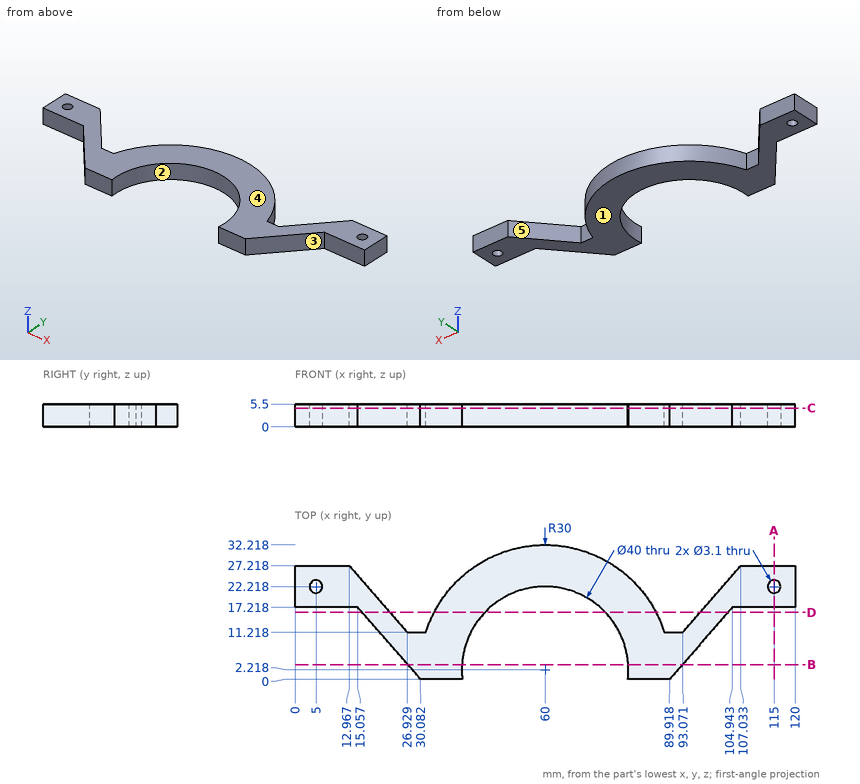
Drawing for the job (mm, zero at the part's lowest x, y, z). A direction names the side the tool comes from. Round coordinates to 2 decimals unless told otherwise and drop trailing zeros. Write each loop counter-clockwise with the first axis right and the second up, starting at its lowest first coordinate (ties: lowest second). Pieces come first, ordered by that corner, then holes. Notation, with made-up numbers: M 83,-21 L 105,-21 A21 ccw 105,7 Z; hole C -15.5,-6.5 d5. An arc over 180 degrees is marked long. One line per question, with ' | ' between items.
1. Cut at A-A on x = 115. Write the cut outline in (y, z).
Working result:
outline: M 17.22,0 L 20.67,0 L 20.67,5.5 L 17.22,5.5 Z; M 23.77,0 L 27.22,0 L 27.22,5.5 L 23.77,5.5 Z
2. Cut at B-B on y = 3.5. Write the cut outline in (x, z), and give its area (3 significant figures).
Working result:
outline: M 27.03,0 L 40.04,0 L 40.04,5.5 L 27.03,5.5 Z; M 79.96,0 L 92.97,0 L 92.97,5.5 L 79.96,5.5 Z | area: 143 mm2
3. Mould opens along X. For the marked faces 1, 2 and 3 say: pulls with the +X half, pulls with the -X half, needs draft (parallel to the pull), parting line crosses it, or undercut.
Working result:
face 1: needs draft | face 2: undercut | face 3: pulls with the +X half
4. Probe L1, parallel to Y at x = 5, z = 2.1; L2, parallel to X at y = 19.5, z = 4.15 (1 decimal); L3, parallel to X at y = 14, z = 0.9 (1 decimal). List the from-to ranges inside material, lowest first. Write a range as from..to.
Working result:
L1: 17.22..20.67, 23.77..27.22 | L2: 0..19.7, 35.5..49.9, 70.1..84.5, 100.3..120 | L3: 17.9..24.5, 32.4..43.8, 76.2..87.6, 95.5..102.1
5. Pin check, flat tips, straight feed: pin 1 Ø1.6 at (x, z) = (115.5, 1.5) entering from -Y; pin 2 Ø3 at (x, y) = (115, 22.22) entering from -Z; pin 3 Ø1.6 at (x, z) = (113.5, 3) entering from +Y; pin 4 Ø1.3 at (x, z) = (30.5, 4) entering from +Y. Stop position of each tip, or through.
Working result:
pin 1: y = 17.22 | pin 2: through | pin 3: y = 27.22 | pin 4: y = 11.22
6. Which spindle directions (+Z, -Z, +X, -X, +Y, -Y) get a long thin tool onto all of the face, cutting with end or side? Do the marked faces 4 and 5. Say none if no direction does.
Working result:
face 4: +Z, +X, -X, +Y, -Y | face 5: +Z, -Z, +Y
7. Cut at C-C on z = 4.5. Write the cut outline in (x, y).
Working result:
outline: M 0,17.22 L 15.06,17.22 L 30.08,0 L 40.12,0 A20 cw long 79.88,0 L 89.92,0 L 104.94,17.22 L 120,17.22 L 120,27.22 L 107.03,27.22 L 93.07,11.22 L 88.62,11.22 A30 ccw 31.38,11.22 L 26.93,11.22 L 12.97,27.22 L 0,27.22 Z; hole C 5,22.22 d3.1; hole C 115,22.22 d3.1
8. Cut at D-D on y = 16. Write the cut outline in (x, z).
Working result:
outline: M 16.12,0 L 22.76,0 L 22.76,5.5 L 16.12,5.5 Z; M 33.35,0 L 45.51,0 L 45.51,5.5 L 33.35,5.5 Z; M 74.49,0 L 86.65,0 L 86.65,5.5 L 74.49,5.5 Z; M 97.24,0 L 103.88,0 L 103.88,5.5 L 97.24,5.5 Z
